```python
from build123d import *

# Parameters (mm, degrees)
CORTAR_EXTRUIR1_REACH   = 7.49
CROQUIS1_R              = 0.225
SALIENTE_EXTRUIR1_DEPTH = 4
CROQUIS2_R              = 0.225
CORTAR_EXTRUIR2_DEPTH   = 1
REDONDEO1_R             = 0.225


with BuildPart() as part:
    # Sketch2 → Revolve1 (revolve)
    with BuildSketch(Plane.XY):
        with BuildLine():
            Line((0, 0), (-1.87, 0))
            Line((-1.87, 0), (-1.87, 1))
            Line((-1.87, 1), (-1.5, 1))
            Line((-1.5, 1), (-1.5, 3.99))
            ThreePointArc((-1.5, 3.99), (-1.060660172, 5.050660172), (0, 5.49))
            Line((0, 5.49), (0, 0))
        make_face()
    revolve(axis=Axis((0, 0, 0), (0, 1, 0)))

    # Sketch3 → Cortar-Extruir1 (cut, up to next)
    with BuildSketch(Plane.XZ, mode=Mode.PRIVATE) as cortar_extruir1_sk1:
        Polygon((1.5, 20.122635641), (1.5, 1.116646766), (1.5, -1.116646766), (1.5, -20.122635641), (39.51197775, -20.122635641), (39.51197775, 20.122635641), align=None)
    cortar_extruir1_tool1 = extrude(cortar_extruir1_sk1.sketch, amount=-CORTAR_EXTRUIR1_REACH, mode=Mode.PRIVATE) & part.part
    add(cortar_extruir1_tool1.solids().sort_by_distance((20.505989, 0, 0))[0], mode=Mode.SUBTRACT)

    # Croquis1 → Saliente-Extruir1 (add)
    with BuildSketch(Plane.XZ):
        with Locations((1.27, 0)):
            Circle(CROQUIS1_R)
        with Locations((-1.27, 0)):
            Circle(CROQUIS1_R)
    extrude(amount=SALIENTE_EXTRUIR1_DEPTH)

    # Croquis2 → Cortar-Extruir2 (cut)
    with BuildSketch(Plane.XZ.offset(4)):
        with Locations((1.27, 0)):
            Circle(CROQUIS2_R)
    extrude(amount=-CORTAR_EXTRUIR2_DEPTH, mode=Mode.SUBTRACT)

    # Redondeo1
    redondeo1_edges = [part.edges().sort_by_distance(p)[0] for p in [
        (-1.495, -4, 0),
        (1.045, -3, 0),
    ]]
    fillet(redondeo1_edges, radius=REDONDEO1_R)


solid = part.part
```
For this review, take the finished solid that the model builds, in its own axes (mm). Coordinates: 2 decimals unless noted, no trailing zeros. Loops run counter-clockwise (first coordinate to the right, second up) from the corner with the lowest first, then second, coordinate; pieces in that order, holes last. Notation, with made-up numbers: (27, -25.5) -> (38, -25.5) arc R19 cw to (38, -1.5) -> close; hole circle Ø8 at (87.5, 81.25). An arc over 180 degrees is marked (long way). Return JSON: item names as keys, results as strings. Group by question number.
(1) Consider section B-B, the plane z = 0.5. Give the boundary of the cut face in (x, y).
(2) Consider section A-A, the plane x = 0. Give the boundary of the cut face in (y, z), plus the area to 3 significant figures.
(3) For pin 1 Ø1 at (y, z) = (0.5, 1) entering from -X; pin 2 Ø2 at (x, z) = (-1, -1) entering from -Y, all flat-tipped, find the tip position at first contact; note any pin that passes through.
(4) To check wall thickness, follow L1, parallel to Y at x = 1.15, z = -1.4; L2, parallel to X at y = -1.75, z = -0.1; L3, parallel to X at y = 2, z = -0.05. State the ranges of each line that lie inside material, in increasing order.
(5) Mouldability with a two-part tool opening along Y and no side actions: class faces 1 (the cylindrical face through (1.5, 2.52, 0.07)), 2 (the flat face through (0, 0, 0)) as pulls with the +Y half, pulls with the -Y half, needs draft (parallel to the pull), parting line crosses it, or undercut.
(6) Consider section D-D, the plane y = 2.25. Give the boundary of the cut face in (x, z), plus the area to 3 significant figures.
(7) Consider section C-C, the plane y = 0.25. Give the boundary of the cut face in (x, z).
Results below:
{
 "1": {"outline": "(-1.8, 0) -> (1.5, 0) -> (1.5, 1) -> (1.41, 1) -> (1.41, 3.99) arc R1.41 ccw to (-1.41, 3.99) -> (-1.41, 1) -> (-1.8, 1) -> close"},
 "2": {"outline": "(0, -1.87) -> (1, -1.87) -> (1, -1.5) -> (3.99, -1.5) arc R1.5 ccw to (3.99, 1.5) -> (1, 1.5) -> (1, 1.87) -> (0, 1.87) -> close", "area": "16.2 mm2"},
 "3": {"pin 1": "stops at x = -1.8", "pin 2": "stops at y = -4"},
 "4": {"L1": "y = 0 to 1", "L2": "x = -1.47 to -1.07, 1.07 to 1.47", "L3": "x = -1.5 to 1.5"},
 "5": {"face 1": "needs draft", "face 2": "pulls with the -Y half"},
 "6": {"outline": "circle Ø3 at (0, 0)", "area": "7.07 mm2"},
 "7": {"outline": "(1.5, -1.12) -> (1.5, 1.12) arc R1.87 ccw (long way) to start"}
}
